Geometry check sheet. Reference: the model listing, model coordinates, mm. A direction names the side the tool comes from. Give positions to 0.01 mm unless a question says otherwise; leave off trailing zeros. Loops run counter-clockwise (first coordinate to the right, second up) from the corner with the lowest first, then second, coordinate; pieces in that order, holes last. Notation, with made-up numbers: (66.25, -11.5) -> (124.25, -11.5) arc R23 cw to (124.25, 13.5) -> close; hole circle Ø7 at (-37, 62.5). An arc over 180 degrees is marked (long way). Answer as a JSON object with one key per item and string values.
from build123d import *

# Parameters (mm, degrees)
SKETCH1_R           = 5
BOSS_EXTRUDE1_DEPTH = 2.7
SKETCH2_R           = 4
BOSS_EXTRUDE2_DEPTH = 0.7
FILLET1_R           = 0.4
SKETCH3_W           = 6.5
SKETCH3_H           = 4.5
BOSS_EXTRUDE3_DEPTH = 4.8


with BuildPart() as part:
    # Sketch1 → Boss-Extrude1 (new body)
    with BuildSketch(Plane(origin=(0, 0, 0), x_dir=(1, 0, 0), z_dir=(0, 1, 0))):
        with Locations(Location((0, 0, 0), (0, 0, 90))):
            Circle(SKETCH1_R)
    extrude(amount=BOSS_EXTRUDE1_DEPTH)

    # Sketch2 → Boss-Extrude2 (add)
    with BuildSketch(Plane(origin=(0, 2.7, 0), x_dir=(1, 0, 0), z_dir=(0, 1, 0))):
        with Locations(Location((0, 0, 0), (0, 0, 270))):
            Circle(SKETCH2_R)
    extrude(amount=BOSS_EXTRUDE2_DEPTH)

    # Fillet1
    fillet1_edges = [part.edges().sort_by_distance(p)[0] for p in [
        (0, 3.4, -4),
    ]]
    fillet(fillet1_edges, radius=FILLET1_R)

    # Sketch3 → Boss-Extrude3 (add)
    with BuildSketch(Plane.XZ):
        Rectangle(SKETCH3_W, SKETCH3_H)
    extrude(amount=BOSS_EXTRUDE3_DEPTH)


solid = part.part
1) Section check A-A on z = 0. Record the cut outline in (x, y), plus the area to 3 significant figures.
Geometry check:
{"outline": "(-5, 0) -> (-3.25, 0) -> (-3.25, -4.8) -> (3.25, -4.8) -> (3.25, 0) -> (5, 0) -> (5, 2.7) -> (4, 2.7) -> (4, 3) arc R0.4 ccw to (3.6, 3.4) -> (-3.6, 3.4) arc R0.4 ccw to (-4, 3) -> (-4, 2.7) -> (-5, 2.7) -> close", "area": "63.7 mm2"}
2) Section check C-C on y = -1.25. Record the cut outline in (x, z).
Geometry check:
{"outline": "(-3.25, -2.25) -> (3.25, -2.25) -> (3.25, 2.25) -> (-3.25, 2.25) -> close"}
3) Section check B-B on x = 0. Record the cut outline in (y, z).
Geometry check:
{"outline": "(-4.8, -2.25) -> (0, -2.25) -> (0, -5) -> (2.7, -5) -> (2.7, -4) -> (3, -4) arc R0.4 ccw to (3.4, -3.6) -> (3.4, 3.6) arc R0.4 ccw to (3, 4) -> (2.7, 4) -> (2.7, 5) -> (0, 5) -> (0, 2.25) -> (-4.8, 2.25) -> close"}
4) Tool access check on faces 1 (the face through (3.25, -2, 0)), 2 (the face through (-3.25, -2, 0)), 3 (the face through (0, -2, -2.25)). Record the directions out of +Z, -Z, +X, -X, +Y, -Y that give a thin tool (end or side, any length) a straight path to the whole face; none if there is none.
Geometry check:
{"face 1": "+Z, -Z, +X, -Y", "face 2": "+Z, -Z, -X, -Y", "face 3": "-Z, +X, -X, -Y"}
5) Depth check by flat-ended pin: P1, Ø2, axis at y = -3.5, z = 0.5, coming from the +X side; P2, Ø1.4, axis at x = 0.5, y = -3.5, coming from the +Z side; P3, Ø1.3, axis at y = -1.5, z = 0, coming from the -X side. Enter the tip coordinate at first touch or a pass-through.
Geometry check:
{"P1": "stops at x = 3.25", "P2": "stops at z = 2.25", "P3": "stops at x = -3.25"}
6) Material ranges on line 1 along Y through (x, z) = (-2, 3); line 2 along Y through (x, z) = (-3.25, 3.25); line 3 along X through (y, z) = (1.25, -3), recorded low to high. Write a range as from..to.
Geometry check:
{"line 1": "y = 0..3.4", "line 2": "y = 0..2.7", "line 3": "x = -4..4"}
7) Section check D-D on y = 2. Record the cut outline in (x, z), plus the area to 3 significant figures.
Geometry check:
{"outline": "circle Ø10 at (0, 0)", "area": "78.5 mm2"}
